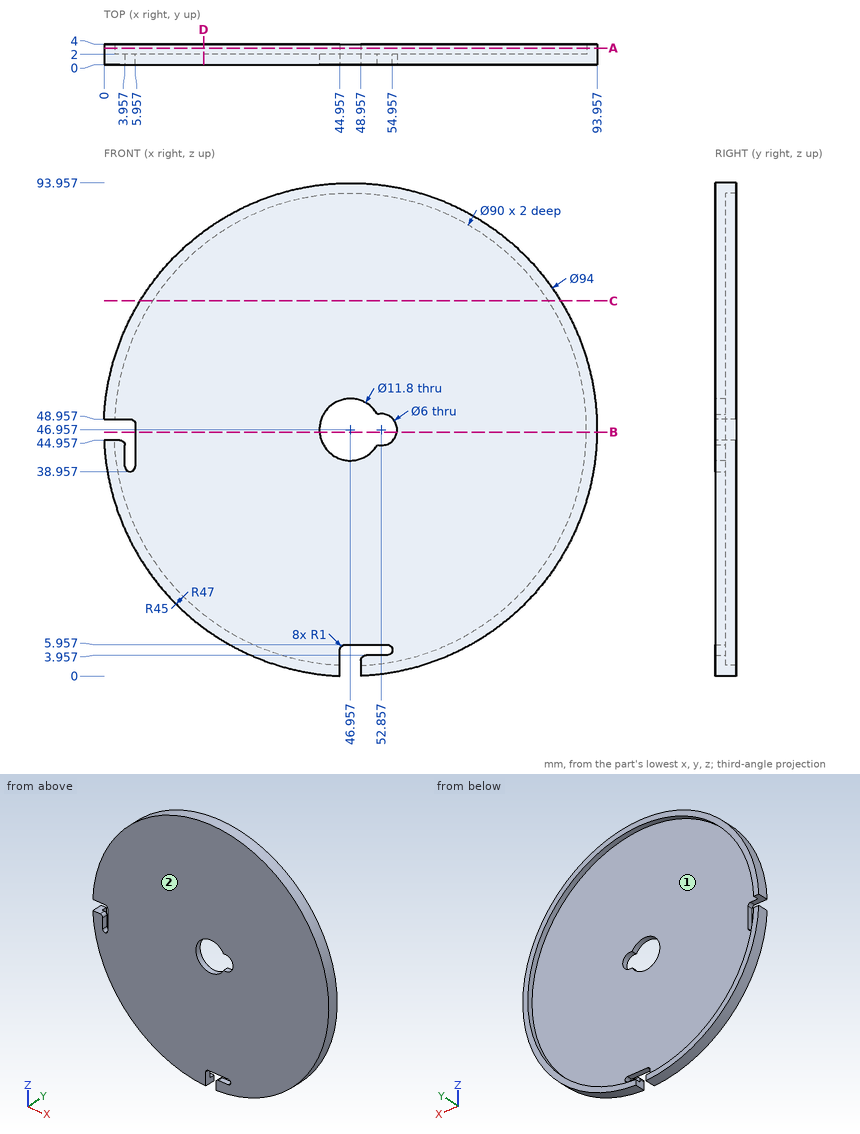
The figure shows three views and two pictorial views of one solid part (mm, origin at its lowest corner). Answer the questions. Coordinates: 2 decimals unless noted, no trailing zeros. Write each loop counter-clockwise with the first axis right and the second up, starting at its lowest first coordinate (ties: lowest second). Pieces come first, ordered by that corner, then holes. Notation, with made-up numbers: (-8.75, 44) -> (27.25, 44) arc R18 ccw to (27.25, 70) -> close; hole circle Ø6 at (-38.5, 33). An arc over 180 degrees is marked (long way). Return JSON: item names as keys, results as strings.
1. Determine the mould class of the marked faces 1 and 2 for opening direction Z: pulls with the +Z half, pulls with the -Z half, needs draft (parallel to the pull), parting line crosses it, or undercut.
Found:
{"face 1": "undercut", "face 2": "needs draft"}
2. A cutting plane is placed at B-B (z = 46.5). Determine the outline of the cut face in (x, y) (1 decimal).
Found:
{"outline": "(6, 0) -> (41.1, 0) -> (41.1, 2) -> (6, 2) -> close; (55.8, 0) -> (94, 0) -> (94, 4) -> (92, 4) -> (92, 2) -> (55.8, 2) -> close"}
3. A cutting plane is placed at C-C (z = 71.5). Determine the outline of the cut face in (x, y) (1 decimal), and give its area (3 significant figures).
Found:
{"outline": "(6.9, 0) -> (87, 0) -> (87, 4) -> (84.7, 4) -> (84.7, 2) -> (9.2, 2) -> (9.2, 4) -> (6.9, 4) -> close", "area": "170 mm2"}
4. A cutting plane is placed at A-A (y = 3.2). Determine the outline of the cut face in (x, z).
Found:
{"outline": "(0, 44.96) arc R47 ccw to (44.96, 0) -> (44.96, 2) arc R45 cw to (2, 44.96) -> close; (0, 48.96) -> (2, 48.96) arc R45 cw (long way) to (48.96, 2) -> (48.96, 0) arc R47 ccw (long way) to start"}
5. Each of these flat-tipped pins is pushed along its axis until it touches: P1, Ø1, axis at y = 3, z = 57.5, coming from the +X side; P2, Ø1, axis at y = 3, z = 60.5, coming from the -X side; P3, Ø8, axis at x = 34.5, z = 69, coming from the +Y side. Where does it stop, or does it pass through?
Found:
{"P1": "x = 92.87", "P2": "x = 1.8", "P3": "y = 2"}
6. Find the intervals of material crossed by line 1 along Y through (x, z) = (64.5, 29); line 2 along Z through (x, y) = (45.5, 2.5) (1 decimal); line 3 along X through (y, z) = (2.4, 59.5) (1 decimal), in increasing order. Write a range as from..to.
Found:
{"line 1": "0..2", "line 2": "91.9..93.9", "line 3": "1.7..3.7, 90.2..92.3"}
7. A cutting plane is placed at D-D (x = 19). Determine the outline of the cut face in (y, z) (1 decimal).
Found:
{"outline": "(0, 9.2) -> (4, 9.2) -> (4, 11.7) -> (2, 11.7) -> (2, 82.2) -> (4, 82.2) -> (4, 84.7) -> (0, 84.7) -> close"}
